Autodesk Inventor part; units mm, degrees
ref_plane "YZ Plane" through (0, 0, 0) normal (1, 0, 0) x (0, 1, 0)
ref_plane "XZ Plane" through (0, 0, 0) normal (0, 1, 0) x (-1, 0, 0)
ref_plane "XY Plane" through (0, 0, 0) normal (0, 0, 1) x (1, 0, 0)
sketch "스케치1" plane through (0, 0, 0) normal (0, 1, 0) x (-1, 0, 0)
  line L0 (7.5, 7.5) -> (-7.5, 7.5)
  line L1 (-7.5, 7.5) -> (-7.5, -7.5)
  line L2 (-7.5, -7.5) -> (7.5, -7.5)
  line L3 (7.5, -7.5) -> (7.5, 7.5)
  line L4 (7.5, 7.5) -> (-7.5, -7.5) construction
  line L5 (-7.5, 7.5) -> (7.5, -7.5) construction
  point P0 (0, 0)
  dimension "d0" = 15
  dimension "d1" = 15
extrude "돌출1" add sketch "스케치1" along normal blind 7
sketch "스케치2" plane through (-7.5, 0, 7.5) normal (0, 0, 1) x (1, 0, 0)
  circle A0 centre (7.5, 3.5) radius 2.5
  line L0 (0, 0) -> (15, 0)
  line L1 (0, 0) -> (0, 7)
  line L2 (5.5, 5) -> (9.5, 5)
  point P0 (7.5, 0)
  point P1 (7.5, 0)
  point P2 (0, 3.5)
  dimension "d5" = 5
  dimension "d14" = 1.5
chamfer "모따기1" distance 0.5 angle 45 8 edges at (0, 7, 7.5) (0, 0, 7.5) (7.5, 0, 0) (0, 0, -7.5) (-7.5, 0, 0) (-7.5, 7, 0) (0, 7, -7.5) (7.5, 7, 0)
extrude "돌출2" cut sketch "스케치2" against normal blind 3 contours A0 L2 picked at (8.1934, 3.1923)
pattern_circular "원형 패턴1" count 4 over 360 about axis through (0, -10, 0) along (0, 1, 0) of "돌출2"
properties part number "몸통"
Can you work these out from the model? Positions are in its coordinate system, mm. A direction names the side the tool comes from. Give positions to 0.01 mm unless a question says otherwise; leave off trailing zeros. Order: outer loops, then holes, each group sorted by start corner. A loop starts at its lowest first (then second) coordinate and runs counter-clockwise, first axis right, second up. Notation, with made-up numbers: (59.5, -38) - (74.5, -38) arc R22 cw to (74.5, -15) - close; hole circle Ø6 at (-32.75, 58.5). An arc over 180 degrees is marked (long way). Use a Markdown table: item, result. Add a question column.
Q1. If we section it at D-D on z = 0: Write out the boundary of the cut face in (x, y).
Q2. If we section it at C-C on x = 0: Write out the boundary of the cut face in (y, z), plus the area to 3 significant figures.
Q3. Please list where these lines run through material, in increasing order: line 1 along Y through (x, z) = (6.85, 0); line 2 along Z through (x, y) = (-6.7, 3.5).
Q4. On a 3-axis mill with a long thin cutter (end or side, diameter ignored), from which of +Z, -Z, +X, -X, +Y, -Y can I reach the whole of each face in a straight line? I mean faces 1 (the flat face through (7.5, 5.5, 0.1)), 2 (the flat face through (4.5, 3, 0)), 3 (the flat face through (-6, 5, 0)), 4 (the cylindrical face through (0, 1, -6)), 5 (the flat face through (0, 5, 6)). Say none if no direction works.
Q5. If we mould it in two halves opening along X, with no side actions, what happens to faces 6 (the flat face through (0, 3, -4.5)), 7 (the flat face through (0.1, 5.5, -7.5)), 8 (the flat face through (-4.5, 3, 0)), 9 (the flat face through (0, 5, -6))? For each: released by +X, released by -X, zero draft, split by the parting line, or undercut.
Q6. If we section it at B-B on y = 3.5: Write out the boundary of the cut face in (x, z).
Q7. I'm going to push flat-ended pins straight in: pin 1 (2 mm diameter, centred on x = 0, y = 3, fed in from +Z); pin 2 (1.2 mm diameter, centred on x = 1, y = 2, fed in from -Z). Where does each tip first touch, or does it pass through?
Q8. If we section it at A-A on z = -5.25: Write out the boundary of the cut face in (x, y), plus the area to 3 significant figures.
Answers follow:
| question | item | result |
|---|---|---|
| 1 | outline | (-7.5, 0.5) - (-7, 0) - (7, 0) - (7.5, 0.5) - (7.5, 1) - (4.5, 1) - (4.5, 5) - (7.5, 5) - (7.5, 6.5) - (7, 7) - (-7, 7) - (-7.5, 6.5) - (-7.5, 5) - (-4.5, 5) - (-4.5, 1) - (-7.5, 1) - close |
| 2 | outline | (0, -7) - (0.5, -7.5) - (1, -7.5) - (1, -4.5) - (5, -4.5) - (5, -7.5) - (6.5, -7.5) - (7, -7) - (7, 7) - (6.5, 7.5) - (5, 7.5) - (5, 4.5) - (1, 4.5) - (1, 7.5) - (0.5, 7.5) - (0, 7) - close |
| 2 | area | 80.5 mm^2 |
| 3 | line 1 | y = 0 to 1, 5 to 7 |
| 3 | line 2 | z = -7.5 to -2.5, 2.5 to 7.5 |
| 4 | face 1 | +Z, -Z, +X, +Y, -Y |
| 4 | face 2 | +X |
| 4 | face 3 | -X |
| 4 | face 4 | -Z |
| 4 | face 5 | +Z |
| 5 | face 6 | undercut |
| 5 | face 7 | zero draft |
| 5 | face 8 | released by -X |
| 5 | face 9 | undercut |
| 6 | outline | (-7.5, -7.5) - (-2.5, -7.5) - (-2.5, -4.5) - (2.5, -4.5) - (2.5, -7.5) - (7.5, -7.5) - (7.5, -2.5) - (4.5, -2.5) - (4.5, 2.5) - (7.5, 2.5) - (7.5, 7.5) - (2.5, 7.5) - (2.5, 4.5) - (-2.5, 4.5) - (-2.5, 7.5) - (-7.5, 7.5) - (-7.5, 2.5) - (-4.5, 2.5) - (-4.5, -2.5) - (-7.5, -2.5) - close |
| 7 | pin 1 | stops at z = 4.5 |
| 7 | pin 2 | stops at z = -4.5 |
| 8 | outline | (-7.5, 0.5) - (-7, 0) - (7, 0) - (7.5, 0.5) - (7.5, 6.5) - (7, 7) - (-7, 7) - (-7.5, 6.5) - close; hole (-2, 5) arc R2.5 ccw (long way) to (2, 5) - close |
| 8 | area | 87.7 mm^2 |
